from build123d import *

# Parameters (mm, degrees)
SKETCH_1_W          = 6.3
SKETCH_1_H          = 59
SKETCH_1_W_2        = 52.5
SKETCH_1_H_2        = 10
EXTRUDE_1_DEPTH     = 4
SKETCH_2_W          = 6.3
SKETCH_2_H          = 4
EXTRUDE_2_DEPTH     = 12.1
SKETCH_3_W          = 6.3
SKETCH_3_H          = 3.4
EXTRUDE_3_DEPTH     = 11
SKETCH_4_W          = 6.3
SKETCH_4_H          = 3.4
EXTRUDE_4_DEPTH     = 11
SKETCH_5_W          = 4
SKETCH_5_H          = 39.574889558
EXTRUDE_5_DEPTH     = 22
SKETCH_6_W          = 2.3
SKETCH_6_H          = 37
CUT_EXTRUDE_1_DEPTH = 89.184238955
FILLET_1_R          = 7
SKETCH_7_W          = 7.91
SKETCH_7_H          = 4
CUT_EXTRUDE_2_DEPTH = 88.542332617
SKETCH_8_W          = 1.9
SKETCH_8_H          = 39.574889558
SKETCH_8_H_2        = 37.097175278
EXTRUDE_6_DEPTH     = 12.7
SKETCH_9_W          = 3
SKETCH_9_H          = 39.574889558
EXTRUDE_7_DEPTH     = 3.5
SKETCH_10_W         = 3
SKETCH_10_H         = 37.097175278
EXTRUDE_8_DEPTH     = 3.5


with BuildPart() as part:
    # Эскиз1 → Бобышка-Вытянуть1 (new body)
    with BuildSketch(Plane.XY):
        with Locations((3.15, 39.5)):
            Rectangle(SKETCH_1_W, SKETCH_1_H)
        with Locations((26.25, 5)):
            Rectangle(SKETCH_1_W_2, SKETCH_1_H_2)
        with Locations((49.35, 39.5)):
            Rectangle(SKETCH_1_W, SKETCH_1_H)
    extrude(amount=EXTRUDE_1_DEPTH)

    # Эскиз2 → Бобышка-Вытянуть2 (add)
    with BuildSketch(Plane.XY.offset(4)):
        with Locations((3.15, 67)):
            Rectangle(SKETCH_2_W, SKETCH_2_H)
        with Locations((49.35, 67)):
            Rectangle(SKETCH_2_W, SKETCH_2_H)
    extrude(amount=EXTRUDE_2_DEPTH)

    # Эскиз3 → Бобышка-Вытянуть3 (add)
    with BuildSketch(Plane.XZ.offset(-65)):
        with Locations((49.35, 14.4)):
            Rectangle(SKETCH_3_W, SKETCH_3_H)
    extrude(amount=EXTRUDE_3_DEPTH)

    # Эскиз4 → Бобышка-Вытянуть4 (add)
    with BuildSketch(Plane.XZ.offset(-65)):
        with Locations((3.15, 14.4)):
            Rectangle(SKETCH_4_W, SKETCH_4_H)
    extrude(amount=EXTRUDE_4_DEPTH)

    # Эскиз5 → Бобышка-Вытянуть5 (add)
    with BuildSketch(Plane.ZY):
        with Locations((2, 27.309730499)):
            Rectangle(SKETCH_5_W, SKETCH_5_H)
    extrude(amount=EXTRUDE_5_DEPTH)

    # Эскиз6 → Вырез-Вытянуть1 (cut, through all)
    with BuildSketch(Plane(origin=(0, 0, 0), x_dir=(-1, 0, 0), z_dir=(0, 0, -1))):
        with Locations((1.15, 30.7)):
            Rectangle(SKETCH_6_W, SKETCH_6_H)
        with Locations((16.15, 30.7)):
            Rectangle(SKETCH_6_W, SKETCH_6_H)
    extrude(amount=-CUT_EXTRUDE_1_DEPTH, mode=Mode.SUBTRACT)

    # Скругление1
    fillet_1_edges = [part.edges().sort_by_distance(p)[0] for p in [
        (0, 7.52228572, 2),
    ]]
    fillet(fillet_1_edges, radius=FILLET_1_R)

    # Эскиз7 → Вырез-Вытянуть2 (cut, through all)
    with BuildSketch(Plane.XY.offset(4)):
        with Locations((29.837829831, 5.560133135)):
            Rectangle(SKETCH_7_W, SKETCH_7_H)
    extrude(amount=-CUT_EXTRUDE_2_DEPTH, mode=Mode.SUBTRACT)

    # Эскиз8 → Бобышка-Вытянуть6 (add)
    with BuildSketch(Plane.XY.offset(4)):
        with Locations((-21.05, 27.309730499)):
            Rectangle(SKETCH_8_W, SKETCH_8_H)
        with Locations((0.95, 28.548587639)):
            Rectangle(SKETCH_8_W, SKETCH_8_H_2)
    extrude(amount=-EXTRUDE_6_DEPTH)

    # Эскиз9 → Бобышка-Вытянуть7 (add)
    with BuildSketch(Plane(origin=(-20.1, 0, 0), x_dir=(0, 0, -1), z_dir=(1, 0, 0))):
        with Locations((7.2, 27.309730499)):
            Rectangle(SKETCH_9_W, SKETCH_9_H)
    extrude(amount=EXTRUDE_7_DEPTH)

    # Эскиз10 → Бобышка-Вытянуть8 (add)
    with BuildSketch(Plane.ZY):
        with Locations((-7.2, 28.548587639)):
            Rectangle(SKETCH_10_W, SKETCH_10_H)
    extrude(amount=EXTRUDE_8_DEPTH)


solid = part.part
Could you check a few things on this model? Use its own coordinates, in mm. A direction names the side the tool comes from. Coordinates: 2 decimals unless noted, no trailing zeros. Write each loop counter-clockwise with the first axis right and the second up, starting at its lowest first coordinate (ties: lowest second). Pieces come first, ordered by that corner, then holes. Notation, with made-up numbers: (41, 79.25) - (54, 79.25) arc R20 ccw to (54, 87.25) - close; hole circle Ø11 at (18, -4.75). An arc over 180 degrees is marked (long way). Write item = value, one per line.
1) For faces 4 (the flat face through (26, 10, 2)), 5 (the flat face through (-20.1, 27, -3)), 6 (the flat face through (0.4, 47.097, -5.4)), 7 (the flat face through (-16, 12.2, 2)), 8 (the flat face through (49, 60, 12.7)), which set-ups out of +Z, -Z, +X, -X, +Y, -Y let a thin tool reach every point of the face, with its end or its side?
Result set:
face_4 = +Z, -Z, +Y
face_5 = +Y, -Y
face_6 = -Z, +X, -X, +Y
face_7 = +Z, +Y
face_8 = +X, -X, -Y
2) We'd pull the mould along X, two halves only. Please class faces 1 (the cylindrical face through (-2, 5.42, 2.03)), 2 (the flat face through (3, 65, 8)), 3 (the flat face through (5, 24, 0)): +X half, -X half, draft (parallel to the pull), parting line (faces both ways), or undercut.
Result set:
face_1 = -X half
face_2 = draft
face_3 = undercut
3) Suppose I cut it at D-D on x = 3.5. Please give me the cut outline in (y, z), plus the area to 3 significant figures.
Result set:
outline = (0, 0) - (69, 0) - (69, 16.1) - (54, 16.1) - (54, 12.7) - (65, 12.7) - (65, 4) - (0, 4) - close
area = 362 mm2
4) Please list where these lines run through material, in increasing order: line 1 (X direction, y = 63, z = 2.75); line 2 (X direction, y = 12.5, z = 0.5); line 3 (X direction, y = 36, z = -1). Write a range as [from, to].
Result set:
line_1 = [0, 6.3], [46.2, 52.5]
line_2 = [-22, -17.3], [-15, -2.3], [0, 6.3], [46.2, 52.5]
line_3 = [-22, -20.1], [0, 1.9]
5) Suppose I cut it at A-A on z = -3.5. Please give me the cut outline in (x, y).
Result set:
outline = (-22, 7.52) - (-20.1, 7.52) - (-20.1, 47.1) - (-22, 47.1) - close; (0, 10) - (1.9, 10) - (1.9, 47.1) - (0, 47.1) - close
6) Will these pins go through, and if not, where does the flat tip stop? pin 1 Ø10 at (x, z) = (31.5, -3) entering from +Y; pin 2 Ø10 at (x, z) = (-18, -3.5) entering from -Y; pin 3 Ø3.5 at (x, z) = (51, 15) entering from -Y.
Result set:
pin_1 = 10
pin_2 = 7.52
pin_3 = 54
7) Suppose I cut it at C-C on y = 57. Please give me the cut outline in (x, z).
Result set:
outline = (0, 0) - (6.3, 0) - (6.3, 4) - (0, 4) - close; (0, 12.7) - (6.3, 12.7) - (6.3, 16.1) - (0, 16.1) - close; (46.2, 0) - (52.5, 0) - (52.5, 4) - (46.2, 4) - close; (46.2, 12.7) - (52.5, 12.7) - (52.5, 16.1) - (46.2, 16.1) - close
8) Suppose I cut it at B-B on x = 31.5. Please give me the cut outline in (y, z), plus the area to 3 significant figures.
Result set:
outline = (0, 0) - (3.56, 0) - (3.56, 4) - (0, 4) - close; (7.56, 0) - (10, 0) - (10, 4) - (7.56, 4) - close
area = 24.0 mm2
